```python
from build123d import *

# Parameters (mm, degrees)
SKETCH1_R      = 88.9
SKETCH1_R_2    = 69.85
EXTRUDE1_DEPTH = 25.4
FILLET1_R      = 6.35
SKETCH2_R      = 69.85
SKETCH2_R_2    = 9.525
EXTRUDE2_DEPTH = 0.79375
SKETCH3_R      = 9.525
SKETCH3_R_2    = 4.7625
EXTRUDE3_DEPTH = 30.1625
SKETCH4_R      = 44.45
SKETCH4_R_2    = 42.8625
EXTRUDE4_DEPTH = 12.7


with BuildPart() as part:
    # Sketch1 → Extrude1 (new, symmetric)
    with BuildSketch(Plane.XY):
        Circle(SKETCH1_R)
        Circle(SKETCH1_R_2, mode=Mode.SUBTRACT)
    extrude(amount=EXTRUDE1_DEPTH, both=True)

    # Fillet1
    fillet1_edges = [part.edges().sort_by_distance(p)[0] for p in [
        (-88.9, 0, -25.4),
        (-88.9, 0, 25.4),
    ]]
    fillet(fillet1_edges, radius=FILLET1_R)

    # Sketch2 → Extrude2 (add, symmetric)
    with BuildSketch(Plane.XY):
        Circle(SKETCH2_R)
        Circle(SKETCH2_R_2, mode=Mode.SUBTRACT)
    extrude(amount=EXTRUDE2_DEPTH, both=True)

    # Sketch3 → Extrude3 (add, symmetric)
    with BuildSketch(Plane.XY.offset(0.79375)):
        with Locations(Location((0, 0, 0), (0, 0, 180))):
            Circle(SKETCH3_R)
        with Locations(Location((0, 0, 0), (0, 0, 180))):
            Circle(SKETCH3_R_2, mode=Mode.SUBTRACT)
    extrude(amount=EXTRUDE3_DEPTH, both=True)

    # Sketch4 → Extrude4 (add, symmetric)
    with BuildSketch(Plane.XY.offset(0.79375)):
        Circle(SKETCH4_R)
        Circle(SKETCH4_R_2, mode=Mode.SUBTRACT)
    extrude(amount=EXTRUDE4_DEPTH, both=True)


solid = part.part
```
The listing builds one solid part. Answer for the finished solid, in the listing's coordinates (mm). A direction names the side the tool comes from. Give positions to 0.01 mm unless a question says otherwise; leave off trailing zeros.
1) Determine the mould class of faces 4 (the face through (23.043, 36.142, 7.055)), 5 (the face through (-68, 19, 25.4)), 6 (the face through (84.795, 26.703, 0.267)) for opening direction Y: pulls with the +Y half, pulls with the -Y half, needs draft (parallel to the pull), parting line crosses it, or undercut.
Reported:
face 4: undercut
face 5: needs draft
face 6: parting line crosses it
2) Consider line 1 along Z through (x, y) = (23, -21); line 2 along Z through (x, y) = (1, -78); line 3 along Y through (x, z) = (25, 13). Determine where each line is inside the solid, lowest interval first.
Reported:
line 1: z = -0.79 to 0.79
line 2: z = -25.4 to 25.4
line 3: y = -85.31 to -65.22, -36.75 to -34.82, 34.82 to 36.75, 65.22 to 85.31
3) For faces 1 (the face through (42.397, 13.352, -6.272)), 2 (the face through (2.3, -4.4, 30.956)), 3 (the face through (-23.3, 36.4, 13.494)), determine the directions among +Z, -Z, +X, -X, +Y, -Y from which every point of the face is accessible in a straight line to the end or side of a thin tool.
Reported:
face 1: -Z
face 2: +Z, +X, -X, +Y, -Y
face 3: +Z
4) Find section A-A on z = -7. Give the number of separate pieces and of enclosed holes in the cut face, then the cut area to 4 significant figures.
Reported:
separate pieces: 3
enclosed holes: 3
area: 10,150 mm2
5) Given P1, Ø3, axis at x = 61, z = 18, coming from the +Y side; P2, Ø12.5, axis at x = 0, y = 0, coming from the -Z side; P3, Ø4, axis at x = -36.5, y = -40, coming from the -Z side; P4, Ø6, axis at x = -26.5, z = -20, coming from the -Y side, each flat-ended and moving along its own axis, determine where each tip first touches the part or whether it passes through.
Reported:
P1: stops at y = 66.05
P2: stops at z = -29.37
P3: stops at z = -0.79
P4: stops at y = -85.71
